```python
from build123d import *

# Parameters (mm, degrees)
SKETCH1_R           = 21
SKETCH1_R_2         = 15.4
SKETCH1_R_3         = 10
BOSS_EXTRUDE1_DEPTH = 5
SKETCH2_R           = 1.5
CUT_EXTRUDE1_DEPTH  = 31.116440693
SKETCH1_3_R         = 10
BOSS_EXTRUDE2_DEPTH = 26
CIRPATTERN1_COUNT   = 8
SKETCH1_4_R         = 15.4
SKETCH1_4_R_2       = 10
BOSS_EXTRUDE3_DEPTH = 18
CHAMFER2_SIZE       = 5
SKETCH3_R           = 4.75
BOSS_EXTRUDE4_DEPTH = 30


with BuildPart() as part:
    # Sketch1 → Boss-Extrude1 (new body)
    # profile 1 of 3: a face of its own
    with BuildSketch(Plane.XY):
        Circle(SKETCH1_R)
        Circle(SKETCH1_R_2, mode=Mode.SUBTRACT)
    # profile 2 of 3: a face of its own
    with BuildSketch(Plane.XY):
        Circle(SKETCH1_R_2)
        Circle(SKETCH1_R_3, mode=Mode.SUBTRACT)
    # profile 3 of 3: a face of its own
    with BuildSketch(Plane.XY):
        Circle(SKETCH1_R_3)
    extrude(amount=BOSS_EXTRUDE1_DEPTH)

    # Sketch2 → Cut-Extrude1 (cut, through all)
    with BuildSketch(Plane(origin=(0, 0, 0), x_dir=(-1, 0, 0), z_dir=(0, 0, -1))):
        with Locations((0, 18)):
            Circle(SKETCH2_R)
    cut_extrude1 = extrude(amount=-CUT_EXTRUDE1_DEPTH, mode=Mode.SUBTRACT)

    # Sketch1_3 → Boss-Extrude2 (add)
    with BuildSketch(Plane.XY):
        Circle(SKETCH1_3_R)
    extrude(amount=-BOSS_EXTRUDE2_DEPTH)

    # CirPattern1: Cut-Extrude1 ×8 about axis
    cirpattern1_axis = Axis((0, 0, 0), (0, 0, 1))
    for i in range(1, CIRPATTERN1_COUNT):
        add(cut_extrude1.rotate(cirpattern1_axis, i * 360 / CIRPATTERN1_COUNT), mode=Mode.SUBTRACT)

    # Sketch1_4 → Boss-Extrude3 (add)
    with BuildSketch(Plane.XY):
        Circle(SKETCH1_4_R)
        Circle(SKETCH1_4_R_2, mode=Mode.SUBTRACT)
    extrude(amount=-BOSS_EXTRUDE3_DEPTH)

    # Chamfer2
    chamfer2_edges = [part.edges().sort_by_distance(p)[0] for p in [
        (-15.4, 0, -18),
    ]]
    chamfer(chamfer2_edges, length=CHAMFER2_SIZE)

    # Sketch3 → Boss-Extrude4 (add)
    with BuildSketch(Plane(origin=(0, 0, -26), x_dir=(-1, 0, 0), z_dir=(0, 0, -1))):
        Circle(SKETCH3_R)
    extrude(amount=BOSS_EXTRUDE4_DEPTH)


solid = part.part
```
The model under review builds one solid part; all positions refer to its coordinate system, in mm. A direction names the side the tool comes from. Coordinates: 2 decimals unless noted, no trailing zeros. Order: outer loops, then holes, each group sorted by start corner. A loop starts at its lowest first (then second) coordinate and runs counter-clockwise, first axis right, second up. Notation, with made-up numbers: (31.5, 26.25) -> (57.5, 26.25) arc R35 cw to (57.5, 60.25) -> close; hole circle Ø8 at (3, 16). An arc over 180 degrees is marked (long way). Answer in a Markdown table with one row per item. Add a question column.
Item 1: Mouldability with a two-part tool opening along Y and no side actions: class faces 1 (the cylindrical face through (12.663, -14.227, 2.465)), 2 (the cylindrical face through (-2.192, -4.214, -40.79)), 3 (the flat face through (0, 0, -56)), 4 (the cylindrical face through (13.92, 13.64, 2.46)) as +Y half, -Y half, draft (parallel to the pull), parting line (faces both ways), or undercut.
Item 2: Clearance check with flat-ended pins moving along their axes: pin 1 (2 mm diameter, centred on x = -11, z = -1.5, fed in from -Y); pin 2 (2 mm diameter, centred on x = 6.5, y = -12, fed in from -Z); pin 3 (5 mm diameter, centred on y = -10, z = -22, fed in from -X); pin 4 (2.5 mm diameter, centred on x = 12.73, y = 12.73, fed in from -Z). State where each tip first meets the part, or that it passes through.
Item 3: Machinability: for faces 5 (the cylindrical face through (-3.338, -15.034, -6.409)), 6 (the cylindrical face through (20.03, 6.31, 2.46)), which of the approach directions +Z, -Z, +X, -X, +Y, -Y give a long, thin tool a straight path to every point of the face, cutting with its end or side? Answer none if there is none.
Item 4: To check wall thickness, follow probe 1 along Y at (x, z) = (0, 1); probe 2 along Z at (x, y) = (-1, -16.5); probe 3 along Y at (x, z) = (-18, 2). State the ranges of each line that lie inside material, in increasing order.
Item 5: We need section A-A on y = 0. Write out the cut boundary in (x, z).
Item 6: We need section C-C on y = 18. Write out the cut boundary in (x, z).
Final values:
| question | item | result |
|---|---|---|
| 1 | face 1 | undercut |
| 1 | face 2 | parting line |
| 1 | face 3 | draft |
| 1 | face 4 | undercut |
| 2 | pin 1 | stops at y = -11.71 |
| 2 | pin 2 | stops at z = -15.75 |
| 2 | pin 3 | stops at x = -6.61 |
| 2 | pin 4 | passes through |
| 3 | face 5 | -Z |
| 3 | face 6 | +Z, -Z |
| 4 | probe 1 | y = -21 to -19.5, -16.5 to 16.5, 19.5 to 21 |
| 4 | probe 2 | z = 0 to 5 |
| 4 | probe 3 | y = -10.82 to -1.5, 1.5 to 10.82 |
| 5 | outline | (-21, 0) -> (-19.5, 0) -> (-19.5, 5) -> (-21, 5) -> close; (-16.5, 0) -> (-15.4, 0) -> (-15.4, -13) -> (-10.4, -18) -> (-10, -18) -> (-10, -26) -> (-4.75, -26) -> (-4.75, -56) -> (4.75, -56) -> (4.75, -26) -> (10, -26) -> (10, -18) -> (10.4, -18) -> (15.4, -13) -> (15.4, 0) -> (16.5, 0) -> (16.5, 5) -> (-16.5, 5) -> close; (19.5, 0) -> (21, 0) -> (21, 5) -> (19.5, 5) -> close |
| 6 | outline | (-10.82, 0) -> (-1.5, 0) -> (-1.5, 5) -> (-10.82, 5) -> close; (1.5, 0) -> (10.82, 0) -> (10.82, 5) -> (1.5, 5) -> close |
